Can you work these out from the model? Positions are in its coordinate system, mm. Give positions to 0.01 mm unless a question says otherwise; leave off trailing zeros. Order: outer loops, then holes, each group sorted by start corner. A loop starts at its lowest first (then second) coordinate and runs counter-clockwise, first axis right, second up. Notation, with made-up numbers: (-24, 18) -> (-18, 18) arc R24 ccw to (-18, 45) -> close; hole circle Ø10 at (1, 63.25). An arc over 180 degrees is marked (long way). Answer as CSV lines item,"result".
Autodesk Inventor part; units mm, degrees
ref_plane "YZ Plane" through (0, 0, 0) normal (1, 0, 0) x (0, 1, 0)
ref_plane "XZ Plane" through (0, 0, 0) normal (0, 1, 0) x (-1, 0, 0)
ref_plane "XY Plane" through (0, 0, 0) normal (0, 0, 1) x (1, 0, 0)
sketch "Sketch1" plane through (0, 0, 0) normal (0, 0, 1) x (1, 0, 0)
  line L0 (-21.7703, 20.0792) -> (29.0297, 20.0792)
  line L1 (29.0297, 20.0792) -> (29.0297, -5.3208)
  line L2 (29.0297, -5.3208) -> (-21.7703, -5.3208)
  line L3 (-21.7703, -5.3208) -> (-21.7703, 20.0792)
  dimension "d0" = 25.4
  dimension "d1" = 50.8
extrude "Extrusion1" add sketch "Sketch1" along normal blind 311.15
shell "Shell1" thickness 3.175 removed faces 2 at (-4.8369, 11.6125, 311.15) at (-4.8369, 11.6125, 0)
draft "FaceDraft1" angle 20.6 pull direction (0, -1, 0) faces at (-3.7786, 19.0209, 0) fixed edges at (3.6297, 20.0792, 0)
properties part number "FE-00013-04"
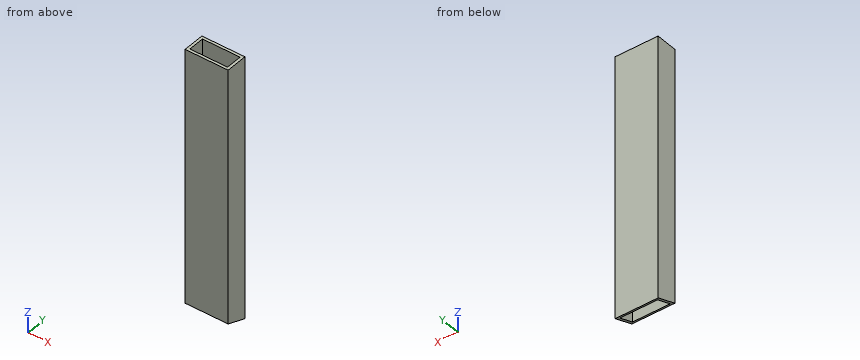
Item 1: Please list where these lines run through material, in increasing order: line 1 along Y through (x, z) = (20.5, 179.5); line 2 along X through (y, z) = (8.5, 113); line 3 along Z through (x, y) = (10, -2.75).
Numbers:
line 1,"y = -5.32 to -2.15, 16.9 to 20.08"
line 2,"x = -21.77 to -18.6, 25.85 to 29.03"
line 3,"z = 8.58 to 311.15"
Item 2: Imagine slicing it at B-B, the plane x = -14. Please give me the cut outline in (y, z).
Numbers:
outline,"(-5.32, 9.55) -> (-2.15, 8.35) -> (-2.15, 311.15) -> (-5.32, 311.15) -> close; (16.9, 1.19) -> (20.08, 0) -> (20.08, 311.15) -> (16.9, 311.15) -> close"
Item 3: Imagine slicing it at C-C, the plane y = 7.5. Please give me the cut outline in (x, z).
Numbers:
outline,"(-21.77, 4.73) -> (-18.6, 4.73) -> (-18.6, 311.15) -> (-21.77, 311.15) -> close; (25.85, 4.73) -> (29.03, 4.73) -> (29.03, 311.15) -> (25.85, 311.15) -> close"
Item 4: Imagine slicing it at A-A, the plane z = 168.5. Please give me the cut outline in (x, y).
Numbers:
outline,"(-21.77, -5.32) -> (29.03, -5.32) -> (29.03, 20.08) -> (-21.77, 20.08) -> close; hole (-18.6, -2.15) -> (25.85, -2.15) -> (25.85, 16.9) -> (-18.6, 16.9) -> close"
Item 5: For pin 1 (8 mm diameter, centred on x = -2.5, y = 5.5, fed in from +Z); pin 2 (4 mm diameter, centred on x = 20, y = 16, fed in from -Z), each with a flat end and sliding along its axis, tell me the tip position at first contact or that it passes through.
Numbers:
pin 1,"passes through"
pin 2,"stops at z = 0.78"
